```python
from build123d import *

# Parameters (mm, degrees)
SKETCH1_R           = 10
BOSS_EXTRUDE1_DEPTH = 23.5
BOSS_EXTRUDE2_START = 23.5
SKETCH1_3_R         = 5
BOSS_EXTRUDE2_DEPTH = 20
BOSS_EXTRUDE3_DEPTH = 47


with BuildPart() as part:
    # Sketch1 → Boss-Extrude1 (new body)
    with BuildSketch(Plane.XY):
        Circle(SKETCH1_R)
    extrude(amount=BOSS_EXTRUDE1_DEPTH)

    # Sketch1<3> → Boss-Extrude2 (add)
    with BuildSketch(Plane.XY.offset(BOSS_EXTRUDE2_START)):
        Circle(SKETCH1_3_R)
    extrude(amount=BOSS_EXTRUDE2_DEPTH)

    # Sketch1<4> → Boss-Extrude3 (add)
    with BuildSketch(Plane.XY):
        with BuildLine():
            ThreePointArc((9.16515139, 4), (9.789063129, 2.043096437), (10, 0))
            Line((10, 0), (37.504998297, 0))
            Line((37.504998297, 0), (54, 0))
            Line((54, 0), (54, 4))
            Line((54, 4), (9.16515139, 4))
        make_face()
    extrude(amount=BOSS_EXTRUDE3_DEPTH)


solid = part.part
```
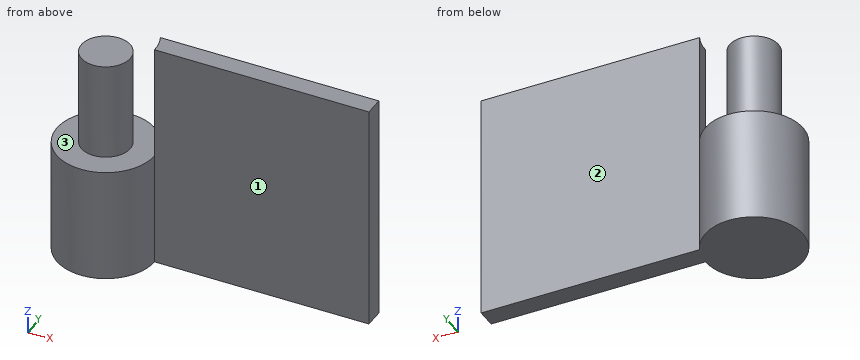
Could you check a few things on this model? Use its own coordinates, in mm. Face numbers are marked on the shaded views. A direction names the side the tool comes from. Give positions to 0.01 mm unless a question says otherwise; leave off trailing zeros. Write each loop counter-clockwise with the first axis right and the second up, starting at its lowest first coordinate (ties: lowest second). Pieces come first, ordered by that corner, then holes. Notation, with made-up numbers: (-25, 30.5) - (7, 30.5) arc R23 ccw to (7, 49.5) - close; hole circle Ø11 at (74.5, 21). An arc over 180 degrees is marked (long way). One line per item, written item: value. Start each with the question number.
Item 1: Imagine slicing it at B-B, the plane x = 0. List the corners of the cut face in (y, z) for me, and give its area (3 significant figures).
Item 2: Please list where these lines run through material, in increasing order: line 1 (Y direction, x = 39, z = 14.5); line 2 (Z direction, x = 3.5, y = 6.25); line 3 (X direction, y = -4.25, z = 24.5). Write a range as from..to.
Item 3: Which directions (+Z, -Z, +X, -X, +Y, -Y) give clear straight access to the entire face, cutting with the end or side of a thin tool? Please do the marked faces 1, 2 and 3.
Item 4: Imagine slicing it at C-C, the plane z = 8. List the corners of the cut face in (x, y) for me.
Item 5: Imagine slicing it at D-D, the plane x = 43. List the corners of the cut face in (y, z) for me.
Item 6: I'm going to push flat-ended pins straight in: pin 1 (8 mm diameter, centred on y = 4.5, z = 31.5, fed in from -X); pin 2 (11 mm diameter, centred on x = 1.5, y = -0.5, fed in from +Z); pin 3 (2 mm diameter, centred on x = 38, z = 12.5, fed in from +Y); pin 4 (1 mm diameter, centred on x = -1.5, y = 3.5, fed in from -Z). Where does each tip first touch, or does it pass through?
Item 7: Imagine slicing it at A-A, the plane z = 29.5. List the corners of the cut face in (x, y) for me, and give its area (3 significant figures).
Geometry says:
1. outline: (-10, 0) - (10, 0) - (10, 23.5) - (5, 23.5) - (5, 43.5) - (-5, 43.5) - (-5, 23.5) - (-10, 23.5) - close
1. area: 670 mm^2
2. line 1: 0..4
2. line 2: 0..23.5
2. line 3: -2.63..2.63
3. face 1: +Z, -Z, +X, -Y
3. face 2: +Z, -Z, +X, +Y
3. face 3: +Z
4. outline: (9.17, 4) arc R10 ccw (long way) to (10, 0) - (54, 0) - (54, 4) - close
5. outline: (0, 0) - (4, 0) - (4, 47) - (0, 47) - close
6. pin 1: x = -4.97
6. pin 2: z = 43.5
6. pin 3: y = 4
6. pin 4: z = 0
7. outline: circle Ø10 at (0, 0); (9.17, 4) arc R10 cw to (10, 0) - (54, 0) - (54, 4) - close
7. area: 256 mm^2
